Check sheet for the modelled part. Datum: model origin and axes. Units: mm. A direction names the side the tool comes from. Coordinates: 2 decimals unless noted, no trailing zeros. Loops run counter-clockwise (first coordinate to the right, second up) from the corner with the lowest first, then second, coordinate; pieces in that order, holes last. Notation, with made-up numbers: (-35, -32) - (-25, -32) arc R14 ccw to (-25, -23) - close; hole circle Ø4 at (-12.5, 16.25). An arc over 180 degrees is marked (long way). Use a Markdown table: item, result. Add a question column.
1) Sectioned sample at A-A, the plane x = 70. Enter the section's corners in (y, z), then the cut area to 3 significant figures.
2) Sectioned sample at B-B, the plane z = 0. Enter the section's corners in (x, y), then the cut area to 3 significant figures.
3) Thickness scan on line 1 (X direction, y = 7.5, z = 15); line 2 (X direction, y = 1.5, z = -17); line 3 (X direction, y = 5.25, z = -8.5). Record the ranges inside material, lowest first.
4) Tool access check on faces 1 (the flat face through (65, 5, 0)), 2 (the flat face through (39, 0, 0)). Record the directions out of +Z, -Z, +X, -X, +Y, -Y that give a thin tool (end or side, any length) a straight path to the whole face; none if there is none.
5) Sectioned sample at C-C, the plane y = 8.5. Enter the section's corners in (x, z).
6) Sectioned sample at D-D, the plane x = 10. Enter the section's corners in (y, z).
7) Draft check along X on faces 3 (the cylindrical face through (68.022, 4.93, 12.421)), 4 (the flat face through (40, 5, -25)), 5 (the flat face through (3, 5, 23)), 6 (the cylindrical face through (11.5, 4.9, -14.6)). Enter one of: pulls with the +X half, pulls with the -X half, needs draft (parallel to the pull), parting line crosses it, or undercut.
from build123d import *

# Parameters (mm, degrees)
SKETCH1_W           = 80
SKETCH1_H           = 50
SKETCH1_R           = 1.75
SKETCH1_R_2         = 11.25
SKETCH1_R_3         = 3.25
BOSS_EXTRUDE1_DEPTH = 10
SKETCH2_R           = 1.5
CUT_EXTRUDE1_DEPTH  = 15
CHAMFER1_SIZE       = 5


with BuildPart() as part:
    # Sketch1 → Boss-Extrude1 (new body)
    with BuildSketch(Plane(origin=(0, 0, 0), x_dir=(1, 0, 0), z_dir=(0, 1, 0))):
        with Locations((40, 0)):
            Rectangle(SKETCH1_W, SKETCH1_H)
        with Locations(Location((10, 15.5, 0), (0, 0, 270))):
            Circle(SKETCH1_R, mode=Mode.SUBTRACT)
        with Locations(Location((10, -15.5, 0), (0, 0, 270))):
            Circle(SKETCH1_R, mode=Mode.SUBTRACT)
        with Locations(Location((25.5, 0, 0), (0, 0, 270))):
            Circle(SKETCH1_R_2, mode=Mode.SUBTRACT)
        with Locations(Location((41, 15.5, 0), (0, 0, 270))):
            Circle(SKETCH1_R, mode=Mode.SUBTRACT)
        with Locations(Location((41, -15.5, 0), (0, 0, 270))):
            Circle(SKETCH1_R, mode=Mode.SUBTRACT)
        with Locations(Location((70, 15, 0), (0, 0, 270))):
            Circle(SKETCH1_R_3, mode=Mode.SUBTRACT)
        with Locations(Location((70, -15, 0), (0, 0, 270))):
            Circle(SKETCH1_R_3, mode=Mode.SUBTRACT)
    extrude(amount=BOSS_EXTRUDE1_DEPTH)

    # Sketch2 → Cut-Extrude1 (cut)
    with BuildSketch(Plane(origin=(80, 0, 0), x_dir=(0, 0, -1), z_dir=(1, 0, 0))):
        with Locations((0, 5)):
            Circle(SKETCH2_R)
    extrude(amount=-CUT_EXTRUDE1_DEPTH, mode=Mode.SUBTRACT)

    # Chamfer1
    chamfer1_edges = [part.edges().sort_by_distance(p)[0] for p in [
        (0, 5, -25),
        (80, 5, -25),
        (80, 5, 25),
        (0, 5, 25),
    ]]
    chamfer(chamfer1_edges, length=CHAMFER1_SIZE)


solid = part.part
Solved:
| question | item | result |
|---|---|---|
| 1 | outline | (0, -25) - (10, -25) - (10, -18.25) - (0, -18.25) - close; (0, -11.75) - (10, -11.75) - (10, 11.75) - (0, 11.75) - close; (0, 18.25) - (10, 18.25) - (10, 25) - (0, 25) - close; hole circle Ø3 at (5, 0) |
| 1 | area | 363 mm2 |
| 2 | outline | (0, 0) - (14.25, 0) - (14.25, 10) - (0, 10) - close; (36.75, 0) - (80, 0) - (80, 3.5) - (65, 3.5) - (65, 6.5) - (80, 6.5) - (80, 10) - (36.75, 10) - close |
| 2 | area | 530 mm2 |
| 3 | line 1 | x = 0 to 8.32, 11.68 to 39.32, 42.68 to 66.75, 73.25 to 80 |
| 3 | line 2 | x = 0 to 9.1, 10.9 to 40.1, 41.9 to 67.44, 72.56 to 80 |
| 3 | line 3 | x = 0 to 18.13, 32.87 to 80 |
| 4 | face 1 | +X |
| 4 | face 2 | +Z, -Z, +X, -X, -Y |
| 5 | outline | (0, -20) - (5, -25) - (75, -25) - (80, -20) - (80, 20) - (75, 25) - (5, 25) - (0, 20) - close; hole circle Ø3.5 at (10, -15.5); hole circle Ø3.5 at (10, 15.5); hole circle Ø22.5 at (25.5, 0); hole circle Ø3.5 at (41, -15.5); hole circle Ø3.5 at (41, 15.5); hole circle Ø6.5 at (70, -15); hole circle Ø6.5 at (70, 15) |
| 6 | outline | (0, -25) - (10, -25) - (10, -17.25) - (0, -17.25) - close; (0, -13.75) - (10, -13.75) - (10, 13.75) - (0, 13.75) - close; (0, 17.25) - (10, 17.25) - (10, 25) - (0, 25) - close |
| 7 | face 3 | undercut |
| 7 | face 4 | needs draft |
| 7 | face 5 | pulls with the -X half |
| 7 | face 6 | undercut |
